from build123d import *

# Parameters (mm, degrees)
BOSS_EXTRUDE1_DEPTH = 9
BOSS_EXTRUDE2_DEPTH = 11.5
BOSS_EXTRUDE3_DEPTH = 18.5
SKETCH3_R           = 2.5
CUT_EXTRUDE1_DEPTH  = 7.5
SKETCH4_R           = 2.75
CUT_EXTRUDE2_DEPTH  = 10
SKETCH4_3_R         = 4.5
SKETCH4_3_R_2       = 2.75
CUT_EXTRUDE3_DEPTH  = 5.5
CIRPATTERN1_COUNT   = 6
SKETCH5_R           = 5
SKETCH5_R_2         = 2.85
CUT_EXTRUDE4_DEPTH  = 2
SKETCH5_2_R         = 2.85
CUT_EXTRUDE5_DEPTH  = 15
SKETCH6_R           = 1
CUT_EXTRUDE6_DEPTH  = 12


with BuildPart() as part:
    # Sketch1 → Boss-Extrude1 (new body)
    with BuildSketch(Plane(origin=(0, 0, 0), x_dir=(1, 0, 0), z_dir=(0, 1, 0))):
        with BuildLine():
            ThreePointArc((-34.794901, -7.040232), (-0.152047, -35.499674), (34.733318, -7.338025))
            Line((34.733318, -7.338025), (22.604769, -7.286078))
            ThreePointArc((22.604769, -7.286078), (-0.101722, -23.749782), (-22.666352, -7.092179))
            Line((-22.666352, -7.092179), (-34.794901, -7.040232))
        make_face()
        with BuildLine():
            Line((34.663333, 7.661812), (22.516948, 7.553114))
            ThreePointArc((22.516948, 7.553114), (-0.21253, 23.749049), (-22.648517, 7.14893))
            Line((-22.648517, 7.14893), (-34.794901, 7.040232))
            ThreePointArc((-34.794901, 7.040232), (-35.5, 0), (-34.794901, -7.040232))
            Line((-34.794901, -7.040232), (-22.666352, -7.092179))
            ThreePointArc((-22.666352, -7.092179), (-0.101722, -23.749782), (22.604769, -7.286078))
            Line((22.604769, -7.286078), (34.733318, -7.338025))
            ThreePointArc((34.733318, -7.338025), (35.307809, -3.688984), (35.5, 0))
            ThreePointArc((35.5, 0), (35.290213, 3.853679), (34.663333, 7.661812))
        make_face()
        with BuildLine():
            ThreePointArc((-22.648517, 7.14893), (-0.21253, 23.749049), (22.516948, 7.553114))
            Line((22.516948, 7.553114), (34.663333, 7.661812))
            ThreePointArc((34.663333, 7.661812), (-0.317676, 35.498579), (-34.794901, 7.040232))
            Line((-34.794901, 7.040232), (-22.648517, 7.14893))
        make_face()
    extrude(amount=-BOSS_EXTRUDE1_DEPTH)

    # Sketch1_3 → Boss-Extrude2 (add)
    with BuildSketch(Plane(origin=(0, 0, 0), x_dir=(1, 0, 0), z_dir=(0, 1, 0))):
        with BuildLine():
            Line((34.663333, 7.661812), (22.516948, 7.553114))
            ThreePointArc((22.516948, 7.553114), (-0.21253, 23.749049), (-22.648517, 7.14893))
            Line((-22.648517, 7.14893), (-34.794901, 7.040232))
            ThreePointArc((-34.794901, 7.040232), (-35.5, 0), (-34.794901, -7.040232))
            Line((-34.794901, -7.040232), (-22.666352, -7.092179))
            ThreePointArc((-22.666352, -7.092179), (-0.101722, -23.749782), (22.604769, -7.286078))
            Line((22.604769, -7.286078), (34.733318, -7.338025))
            ThreePointArc((34.733318, -7.338025), (35.307809, -3.688984), (35.5, 0))
            ThreePointArc((35.5, 0), (35.290213, 3.853679), (34.663333, 7.661812))
        make_face()
    extrude(amount=BOSS_EXTRUDE2_DEPTH)

    # Sketch2 → Boss-Extrude3 (add)
    with BuildSketch(Plane(origin=(0, 11.5, 0), x_dir=(1, 0, 0), z_dir=(0, 1, 0))):
        with BuildLine():
            Line((-4.51754, 19.642857), (-11.293849, 5.357143))
            ThreePointArc((-11.293849, 5.357143), (-12.5, 0), (-11.293849, -5.357143))
            Line((-11.293849, -5.357143), (-4.51754, -19.642857))
            ThreePointArc((-4.51754, -19.642857), (0, -22.5), (4.51754, -19.642857))
            Line((4.51754, -19.642857), (11.293849, -5.357143))
            ThreePointArc((11.293849, -5.357143), (12.5, 0), (11.293849, 5.357143))
            Line((11.293849, 5.357143), (4.51754, 19.642857))
            ThreePointArc((4.51754, 19.642857), (0, 22.5), (-4.51754, 19.642857))
        make_face()
    extrude(amount=BOSS_EXTRUDE3_DEPTH)

    # Sketch3 → Cut-Extrude1 (cut)
    with BuildSketch(Plane(origin=(0, 30, 0), x_dir=(1, 0, 0), z_dir=(0, 1, 0))):
        with Locations((0, 17.465877)):
            Circle(SKETCH3_R)
        with Locations((0, -17.534123)):
            Circle(SKETCH3_R)
    extrude(amount=-CUT_EXTRUDE1_DEPTH, mode=Mode.SUBTRACT)

    # Sketch4 → Cut-Extrude2 (cut, through all)
    with BuildSketch(Plane(origin=(0, 0, 0), x_dir=(1, 0, 0), z_dir=(0, 1, 0))):
        with Locations((0, 29.5)):
            Circle(SKETCH4_R)
    cut_extrude2 = extrude(amount=-CUT_EXTRUDE2_DEPTH, mode=Mode.SUBTRACT)

    # Sketch4_3 → Cut-Extrude3 (cut)
    with BuildSketch(Plane(origin=(0, 0, 0), x_dir=(1, 0, 0), z_dir=(0, 1, 0))):
        with Locations((0, 29.5)):
            Circle(SKETCH4_3_R)
        with Locations((0, 29.5)):
            Circle(SKETCH4_3_R_2, mode=Mode.SUBTRACT)
    cut_extrude3 = extrude(amount=-CUT_EXTRUDE3_DEPTH, mode=Mode.SUBTRACT)

    # CirPattern1: Cut-Extrude2, Cut-Extrude3 ×6 about axis
    cirpattern1_axis = Axis((0, 0, 0), (0, 1, 0))
    for i in range(1, CIRPATTERN1_COUNT):
        add(cut_extrude2.rotate(cirpattern1_axis, i * 360 / CIRPATTERN1_COUNT), mode=Mode.SUBTRACT)
        add(cut_extrude3.rotate(cirpattern1_axis, i * 360 / CIRPATTERN1_COUNT), mode=Mode.SUBTRACT)

    # Sketch5 → Cut-Extrude4 (cut)
    with BuildSketch(Plane(origin=(35.5, 0, 0), x_dir=(0, 0, -1), z_dir=(1, 0, 0))):
        Circle(SKETCH5_R)
        Circle(SKETCH5_R_2, mode=Mode.SUBTRACT)
    cut_extrude4 = extrude(amount=-CUT_EXTRUDE4_DEPTH, mode=Mode.SUBTRACT)

    # Sketch5_2 → Cut-Extrude5 (cut)
    with BuildSketch(Plane(origin=(35.5, 0, 0), x_dir=(0, 0, -1), z_dir=(1, 0, 0))):
        Circle(SKETCH5_2_R)
    cut_extrude5 = extrude(amount=-CUT_EXTRUDE5_DEPTH, mode=Mode.SUBTRACT)

    # Mirror1: Cut-Extrude4, Cut-Extrude5 across plane
    add(cut_extrude4.mirror(Plane(origin=(0, 0, 0), x_dir=(0, 0, 1), z_dir=(1, 0, 0))), mode=Mode.SUBTRACT)
    add(cut_extrude5.mirror(Plane(origin=(0, 0, 0), x_dir=(0, 0, 1), z_dir=(1, 0, 0))), mode=Mode.SUBTRACT)

    # Sketch6 → Cut-Extrude6 (cut)
    with BuildSketch(Plane(origin=(0, 11.5, 0), x_dir=(1, 0, 0), z_dir=(0, 1, 0))):
        with Locations((23, 0)):
            Circle(SKETCH6_R)
    cut_extrude6 = extrude(amount=-CUT_EXTRUDE6_DEPTH, mode=Mode.SUBTRACT)

    # Mirror2: Cut-Extrude6 across plane
    add(cut_extrude6.mirror(Plane(origin=(0, 0, 0), x_dir=(0, 0, 1), z_dir=(1, 0, 0))), mode=Mode.SUBTRACT)

    # Sketch7 → Cut-Revolve1 (revolve, cut)
    with BuildSketch(Plane(origin=(0, 0, 0), x_dir=(0, 0, -1), z_dir=(1, 0, 0))):
        Polygon((0, 30), (0, -9), (-15.5, -9), (-15.5, 0), (-13.133679, 0), (-10.94223, 8.178598), (-7.332377, 8.178598), (-7.332377, 11.5), (-11.5, 11.5), (-11.5, 30), align=None)
    revolve(axis=Axis((0, 30, 0), (0, -1, 0)), mode=Mode.SUBTRACT)


solid = part.part
Source: CAD feature listing. Evaluate the final solid. Frame: model axes, mm. A direction names the side the tool comes from. Round coordinates to 2 decimals unless told otherwise and drop trailing zeros. Order: outer loops, then holes, each group sorted by start corner. A loop starts at its lowest first (then second) coordinate and runs counter-clockwise, first axis right, second up. Notation, with made-up numbers: (48.25, 72.5) -> (79.25, 72.5) arc R30 ccw to (79.25, 108.5) -> close; hole circle Ø7 at (69, -15). An arc over 180 degrees is marked (long way). Answer as CSV lines item,"result".
Item 1: Pull-direction query (X, two-part tool) for faces 4 (the face through (7.86, 20.62, 12.6)), 5 (the face through (15, -9, 7)), 6 (the face through (-15.368, -4.437, -2.018)); classes: pulls with the +X half, pulls with the -X half, needs draft (parallel to the pull), parting line crosses it, or undercut.
A:
face 4,"pulls with the +X half"
face 5,"needs draft"
face 6,"undercut"
Item 2: Reachability of faces 1 (the face through (23, -5.5, -13)), 2 (the face through (-7.86, 20.62, -12.6)), 3 (the face through (-0.6, 0, -24.6)) from +Z, -Z, +X, -X, +Y, -Y: full face, straight path, thin tool, end or side. Return the list, or none.
A:
face 1,"+Y"
face 2,"-Z, -X, +Y"
face 3,"-Z, +Y"
Item 3: Section C-C, the plane z = 29.5. Return loops of the section in (x, y).
A:
outline,"(-19.75, -9) -> (-2.75, -9) -> (-2.75, -5.5) -> (-4.5, -5.5) -> (-4.5, 0) -> (-19.75, 0) -> close; (2.75, -9) -> (19.75, -9) -> (19.75, 0) -> (4.5, 0) -> (4.5, -5.5) -> (2.75, -5.5) -> close"
Item 4: Section B-B, the plane x = -25.5. Return loops of the section in (y, z).
A:
outline,"(-9, -24.7) -> (0, -24.7) -> (0, -19.25) -> (-5.5, -19.25) -> (-5.5, -17.5) -> (-9, -17.5) -> close; (-9, -12) -> (-5.5, -12) -> (-5.5, -10.25) -> (0, -10.25) -> (0, -7.12) -> (11.5, -7.12) -> (11.5, 7.08) -> (0, 7.08) -> (0, 10.25) -> (-5.5, 10.25) -> (-5.5, 12) -> (-9, 12) -> close; (-9, 17.5) -> (-5.5, 17.5) -> (-5.5, 19.25) -> (0, 19.25) -> (0, 24.7) -> (-9, 24.7) -> close; hole circle Ø5.7 at (0, 0)"
Item 5: Section D-D, the plane x = 0. Count the separate pieces of the cut face and the enclosed holes in it, plus the area to 3 significant figures.
A:
separate pieces,"4"
enclosed holes,"0"
area,"855 mm²"
Item 6: Line query: L1, parallel to Z at x = 0, y = -6.2; L2, parallel to Z at x = 29, y = -3; L3, parallel to Z at x = -26.5, y = -1.5. Output: solid intervals per line, ascending.
A:
L1,"-35.5 to -32.25, -26.75 to -15.5, 15.5 to 26.75, 32.25 to 35.5"
L2,"-20.48 to -17.64, -11.86 to 11.86, 17.64 to 20.48"
L3,"-23.62 to -19.15, -10.35 to -2.42, 2.42 to 10.35, 19.15 to 23.62"
Item 7: Pin query (flat end, axial travel): pin 1 Ø10 at (y, z) = (9, -20) entering from +X; pin 2 Ø4.5 at (y, z) = (-1, -1) entering from +X; pin 3 Ø5 at (x, y) = (13.5, 16) entering from -Z. Return the tip coordinate at first contact, or that it passes through.
A:
pin 1,"x = 18.41"
pin 2,"x = 33.5"
pin 3,"z = -5.98"
Item 8: Section A-A, the plane y = 21.5. Return loops of the section in (x, z).
A:
outline,"(-11.29, -5.36) -> (-4.52, -19.64) arc R5 ccw to (4.52, -19.64) -> (11.29, -5.36) arc R12.5 ccw to (11.29, 5.36) -> (4.52, 19.64) arc R5 ccw to (-4.52, 19.64) -> (-11.29, 5.36) arc R12.5 ccw to start; hole circle Ø23 at (0, 0)"
